Check sheet for the modelled part. Datum: model origin and axes. Units: mm. Face numbers are marked on the shaded views. A direction names the side the tool comes from. Round coordinates to 2 decimals unless told otherwise and drop trailing zeros. Write each loop counter-clockwise with the first axis right and the second up, starting at its lowest first coordinate (ties: lowest second). Pieces come first, ordered by that corner, then holes.
Item 1: Section check C-C, the plane y = 12.7. Record the cut outline in (x, z).
Item 2: Set-up check for the marked faces 1, 2, 3, 4 and 5: record each of +Z, -Z, +X, -X, +Y, -Y from which the full face is reachable in a straight line by a thin tool's end or side.
Item 3: Section check D-D, the plane z = 20.5. Record the cut outline in (x, y), plus the area to 3 significant figures.
Item 4: Section check B-B, the plane z = 0. Record the cut outline in (x, y), plus the area to 3 significant figures.
Item 5: Material ranges on line 1 along X through (y, z) = (12.7, 20); line 2 along Z through (x, y) = (12.5, 22.5); line 3 along X through (y, z) = (2, 9.5), recorded low to high.
Item 6: Release check for a two-part mould opening along X. For the marked faces 6, 7 and 8 record: pulls with the +X half, pulls with the -X half, needs draft (parallel to the pull), parting line crosses it, or undercut.
Item 7: Depth check by flat-ended pin: pin 1 (4 mm diameter, centred on y = 10.5, z = -5, fed in from -X); pin 2 (10 mm diameter, centred on x = 66.5, y = 14, fed in from +Z); pin 3 (4 mm diameter, centred on y = 8.5, z = 6, fed in from +X); pin 4 (3.5 mm diameter, centred on x = -33.274, y = 6.35, fed in from -Z). Enter the tip coordinate at first touch or a pass-through.
Item 8: Section check A-A, the plane y = 19.05. Record the cut outline in (x, z).
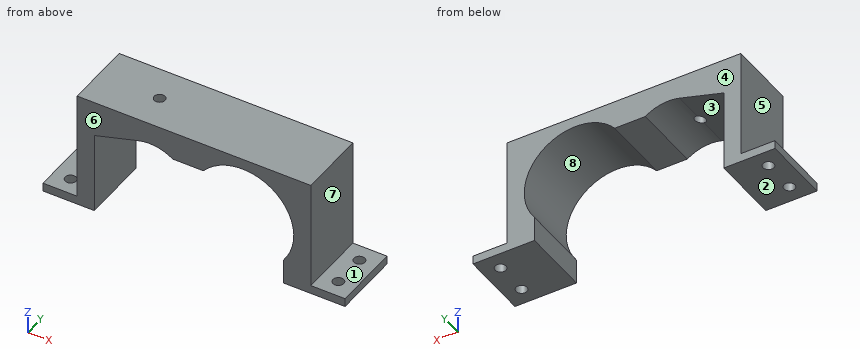
from build123d import *

# Parameters (mm, degrees)
BOSS_EXTRUDE1_DEPTH    = 25.4
SKETCH2_R              = 2.032
CUT_EXTRUDE1_DEPTH     = 87.9904043
F_10_32_TAPPED_HOLE1_D = 4.0386


with BuildPart() as part:
    # Sketch1 → Boss-Extrude1 (new body)
    with BuildSketch(Plane(origin=(0, 0, 0), x_dir=(1, 0, 0), z_dir=(0, 1, 0))):
        with BuildLine():
            Line((-20.574, -9.652129604), (-4.162019583, -14.39674322))
            ThreePointArc((-4.162019583, -14.39674322), (2.459785533, -14.783033433), (8.59971196, -12.273287113))
            Line((8.59971196, -12.273287113), (19.974548279, -12.273287113))
            ThreePointArc((19.974548279, -12.273287113), (46.400384935, -14.910688658), (49.784, 11.43))
            Line((49.784, 11.43), (49.784, 20.746712887))
            Line((49.784, 20.746712887), (72.644, 20.746712887))
            Line((72.644, 20.746712887), (72.644, 17.571712887))
            Line((72.644, 17.571712887), (59.944, 17.571712887))
            Line((59.944, 17.571712887), (59.944, -12.827129604))
            Line((59.944, -12.827129604), (59.944, -22.987129604))
            Line((59.944, -22.987129604), (-26.924, -22.987129604))
            Line((-26.924, -22.987129604), (-26.924, -12.827129604))
            Line((-26.924, -12.827129604), (-26.924, 17.571712887))
            Line((-26.924, 17.571712887), (-39.624, 17.571712887))
            Line((-39.624, 17.571712887), (-39.624, 20.746712887))
            Line((-39.624, 20.746712887), (-20.574, 20.746712887))
            Line((-20.574, 20.746712887), (-20.574, 9.652))
            Line((-20.574, 9.652), (-20.574, -9.652129604))
        make_face()
    extrude(amount=BOSS_EXTRUDE1_DEPTH)

    # Sketch2 → Cut-Extrude1 (cut, through all)
    with BuildSketch(Plane.XY.offset(-17.571712887)):
        with Locations((-33.274, 19.05)):
            Circle(SKETCH2_R)
        with Locations((-33.274, 6.35)):
            Circle(SKETCH2_R)
        with Locations((66.294, 19.05)):
            Circle(SKETCH2_R)
        with Locations((66.294, 6.35)):
            Circle(SKETCH2_R)
    extrude(amount=-CUT_EXTRUDE1_DEPTH, mode=Mode.SUBTRACT)

    # #10-32 Tapped Hole1 (through all)
    with Locations(Plane.XY.offset(22.987129604)):
        with Locations((-4.064, 12.7)):
            Hole(F_10_32_TAPPED_HOLE1_D / 2)


solid = part.part
Values found:
1. outline: (-39.62, -20.75) - (-20.57, -20.75) - (-20.57, 9.65) - (-6.08, 13.84) - (-6.08, 22.99) - (-26.92, 22.99) - (-26.92, -17.57) - (-39.62, -17.57) - close; (-2.04, 14.85) arc R14.99 cw to (8.6, 12.27) - (19.97, 12.27) arc R19.05 cw to (49.78, -11.43) - (49.78, -20.75) - (72.64, -20.75) - (72.64, -17.57) - (59.94, -17.57) - (59.94, 22.99) - (-2.04, 22.99) - close
2. face 1: +Z, +X, +Y, -Y
2. face 2: -Z, +X, -X, +Y, -Y
2. face 3: -Z, +Y, -Y
2. face 4: +Z, -Z, +X, -X, +Y
2. face 5: +Z, -X, +Y, -Y
3. outline: (-26.92, 0) - (59.94, 0) - (59.94, 25.4) - (-26.92, 25.4) - close; hole circle Ø4.04 at (-4.06, 12.7)
3. area: 2,190 mm2
4. outline: (-26.92, 0) - (-20.57, 0) - (-20.57, 25.4) - (-26.92, 25.4) - close; (53.59, 0) - (59.94, 0) - (59.94, 25.4) - (53.59, 25.4) - close
4. area: 323 mm2
5. line 1: x = -26.92 to -6.08, -2.04 to 59.94
5. line 2: z = 12.27 to 22.99
5. line 3: x = -26.92 to -20.57, 51.06 to 59.94
6. face 6: needs draft
6. face 7: pulls with the +X half
6. face 8: undercut
7. pin 1: stops at x = -26.92
7. pin 2: stops at z = -17.57
7. pin 3: stops at x = 59.94
7. pin 4: passes through
8. outline: (-39.62, -20.75) - (-35.31, -20.75) - (-35.31, -17.57) - (-39.62, -17.57) - close; (-31.24, -20.75) - (-20.57, -20.75) - (-20.57, 9.65) - (-4.16, 14.4) arc R14.99 cw to (8.6, 12.27) - (19.97, 12.27) arc R19.05 cw to (49.78, -11.43) - (49.78, -20.75) - (64.26, -20.75) - (64.26, -17.57) - (59.94, -17.57) - (59.94, 22.99) - (-26.92, 22.99) - (-26.92, -17.57) - (-31.24, -17.57) - close; (68.33, -20.75) - (72.64, -20.75) - (72.64, -17.57) - (68.33, -17.57) - close
